Part model, mm, in its own coordinate system. A direction names the side the tool comes from. Coordinates: 2 decimals unless noted, no trailing zeros. Loops run counter-clockwise (first coordinate to the right, second up) from the corner with the lowest first, then second, coordinate; pieces in that order, holes last. Notation, with made-up numbers: (0.5, 79.25) -> (36.5, 79.25) arc R29 cw to (36.5, 100.25) -> close; hole circle Ø10 at (-30.5, 68.5). An arc over 180 degrees is marked (long way). Use one line per item in the form item = value. Start each with the question number.
(1) Mould opens along Z. For faces 3 (the flat face through (-40, 0, 4)), 4 (the cylindrical face through (-44.77, -260.26, 29.58)) say: +Z half, -Z half, draft (parallel to the pull), parting line (faces both ways), or undercut.
(2) Band-saw the part on C-C on z = 2. Give the cut face in (x, y), then the cut area to 3 significant figures.
(3) Band-saw the part on B-B on x = -16.5. Give the cut face in (y, z).
(4) Drill centre lines: L1, parallel to Y at x = -46.5, z = 27.5; L2, parallel to Y at x = -47, z = -15; L3, parallel to X at y = -66.5, z = 2. Where is each one in solid material? Low to high. Write a range as [from, to].
(5) 3-axis set-ups, long thin cutter, end or side, ignore diameter. For faces 1 (the flat face through (-38, -254, 19)), 2 (the flat face through (-45, -266.7, 11)): which of +Z, -Z, +X, -X, +Y, -Y reach the whole face in a straight line?
(6) Band-saw the part on A-A on y = -148.5. Give the cut face in (x, z), then the cut area to 3 significant figures.
(7) Pin check, flat tips, straight feed: P1, Ø10, axis at y = -146.5, z = 34, coming from the +X side; P2, Ø6, axis at x = -36, z = 43.5, coming from the -Y side; P3, Ø12, axis at y = -128.5, z = -5, coming from the -X side. Stop position of each tip, or through.
```python
from build123d import *

# Parameters (mm, degrees)
F0_R     = 25.2255961417
F1_DEPTH = 254
F2_R     = 4.8984695606
F2_R_2   = 4.1135395879
F3_DEPTH = 12.7
F5_DEPTH = 50.8


with BuildPart() as f1:
    # F0 (on Front) → F1 (new body)
    with BuildSketch(Plane.XZ):
        with Locations((-37.837240845, 18.9186204225)):
            Circle(F0_R)
    extrude(amount=F1_DEPTH)

    # F2 (on face) → F3 (join)
    with BuildSketch(Plane.XZ.offset(254)):
        with Locations((-44.693492353, 11.2606054172)):
            Circle(F2_R)
        with Locations((-41.5038913488, 32.080437988)):
            Circle(F2_R_2)
        with BuildLine():
            add(Edge.make_bspline(
                [(-30.9607814997, 22.0860820264), (-31.1174790444, 27.1779190493), (-35.4705043818, 37.384895038), (-19.6123896035, 28.581671559), (-22.3060000408, 13.9240447836), (-29.9356971904, 5.434185596), (-34.1455406145, 8.7707728586), (-30.7894579728, 16.5189783491), (-30.9607814997, 22.0860820264)],
                knots=[0, 0, 0, 0, 0.179844359, 0.3488990719, 0.5500177158, 0.7159973757, 0.8033691597, 1, 1, 1, 1], degree=3))
        make_face()
    extrude(amount=F3_DEPTH)

    # F4 (on Front) → F5 (join)
    with BuildSketch(Plane.XZ):
        with BuildLine():
            add(Edge.make_bspline(
                [(-45.1222844422, 12.1712666005), (-52.9735846355, 16.9556340719), (-64.7701771693, 46.9993806394), (-27.9966636305, 66.0454754857), (-24.6817713236, 14.3898842389), (-39.8118103434, 8.9352090163), (-45.1222844422, 12.1712666005)],
                knots=[0, 0, 0, 0, 0.2823086577, 0.513014559, 0.8090516503, 1, 1, 1, 1], degree=3))
        make_face()
        with BuildLine():
            add(Edge.make_bspline(
                [(-57.3190748692, -10.1838894188), (-54.8526705143, -3.4441726715), (-51.1531019459, 10.2525243726), (-27.5972764056, 9.3930479254), (-18.4794160333, -57.7544605135), (-66.5035831823, -30.9630818541), (-59.7978178724, -16.957322858), (-57.3190748692, -10.1838894188)],
                knots=[0, 0, 0, 0, 0.1765612044, 0.3326258233, 0.6015627152, 0.8225555152, 1, 1, 1, 1], degree=3))
        make_face()
    extrude(amount=F5_DEPTH)


solid = f1.part
```
A:
q1.face_3 = draft
q1.face_4 = undercut
q2.outline = (-56.55, -254) -> (-19.13, -254) -> (-19.13, 0) -> (-56.55, 0) -> close
q2.area = 9,510 mm²
q3.outline = (-254, 5.46) -> (0, 5.46) -> (0, 32.37) -> (-254, 32.37) -> close
q4.L1 = [-254, 0]
q4.L2 = [-50.8, 0]
q4.L3 = [-56.55, -19.13]
q5.face_1 = -Y
q5.face_2 = +Z, -Z, +X, -X, -Y
q6.outline = circle Ø50.45 at (-37.84, 18.92)
q6.area = 2,000 mm²
q7.P1 = -14.71
q7.P2 = -254
q7.P3 = -55.59
